from build123d import *

# Parameters (mm, degrees)
F0_W     = 20
F0_H     = 7
F0_H_2   = 62
F0_W_2   = 16
F0_H_3   = 58
F1_DEPTH = 2
F2_DEPTH = 36
F3_W     = 2
F3_H     = 36
F4_DEPTH = 7
F5_W     = 2
F5_H     = 36
F6_DEPTH = 7
F7_W     = 18
F7_H     = 2
F8_DEPTH = 18


with BuildPart() as f1:
    # F0 (on Top) → F1 (new body)
    with BuildSketch(Plane.XY):
        with Locations((8, 63.5)):
            Rectangle(F0_W, F0_H)
        with Locations((8, 29)):
            Rectangle(F0_W, F0_H_2)
        with Locations((8, 29)):
            Rectangle(F0_W_2, F0_H_3, mode=Mode.SUBTRACT)
        with Locations((8, 29)):
            Rectangle(F0_W_2, F0_H_3)
        with Locations((8, -5.5)):
            Rectangle(F0_W, F0_H)
    extrude(amount=-F1_DEPTH)

    # F0 (on Top) → F2 (join)
    with BuildSketch(Plane.XY):
        with Locations((8, 29)):
            Rectangle(F0_W, F0_H_2)
        with Locations((8, 29)):
            Rectangle(F0_W_2, F0_H_3, mode=Mode.SUBTRACT)
    extrude(amount=F2_DEPTH)

    # F3 (on face) → F4 (join)
    with BuildSketch(Plane.XZ.offset(2)):
        with Locations((-1, 18)):
            Rectangle(F3_W, F3_H)
    extrude(amount=F4_DEPTH)

    # F5 (on face) → F6 (join)
    with BuildSketch(Plane(origin=(0, 60, 0), x_dir=(-1, 0, 0), z_dir=(0, 1, 0))):
        with Locations((1, 18)):
            Rectangle(F5_W, F5_H)
    extrude(amount=F6_DEPTH)

    # F7 (on face) → F8 (cut)
    with BuildSketch(Plane.XY.offset(36)):
        with Locations((9, -1)):
            Rectangle(F7_W, F7_H)
    extrude(amount=-F8_DEPTH, mode=Mode.SUBTRACT)


solid = f1.part
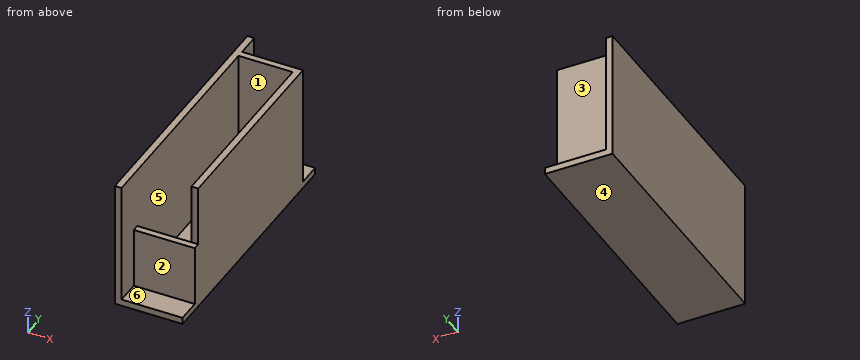
Could you check a few things on this model? Use its own coordinates, in mm. Face numbers are marked on the shaded views. A direction names the side the tool comes from. Round coordinates to 2 decimals unless told otherwise and drop trailing zeros. Write each loop counter-clockwise with the first axis right and the second up, starting at its lowest first coordinate (ties: lowest second). Pieces come first, ordered by that corner, then holes. Notation, with made-up numbers: (3.25, 65.25) - (43.25, 65.25) arc R9 cw to (43.25, 73.25) - close; hole circle Ø3 at (27.25, 68.25). An arc over 180 degrees is marked (long way). Use a Markdown table: item, result.
Q1. Please list where these lines run through material, in increasing order: L1, parallel to X at y = 52, z = 18.5; L2, parallel to Y at x = 7, z = 13; L3, parallel to Y at x = 10.25, z = 19.
Output values:
| item | result |
|---|---|
| L1 | -2 to 0, 16 to 18 |
| L2 | -2 to 0, 58 to 60 |
| L3 | 58 to 60 |
Q2. I want a section at A-A (z = 5.5). List the corners of the cut face in (x, y) for me, plus the area to 3 significant figures.
Output values:
| item | result |
|---|---|
| outline | (-2, -9) - (0, -9) - (0, -2) - (18, -2) - (18, 60) - (0, 60) - (0, 67) - (-2, 67) - close; hole (0, 0) - (16, 0) - (16, 58) - (0, 58) - close |
| area | 340 mm2 |
Q3. Thinking about a two-plate mould opening in Y: for the marked faces 1, 2 and 3, which applies, released by +Y, released by -Y, zero draft, split by the parting line, or undercut?
Output values:
| item | result |
|---|---|
| face 1 | undercut |
| face 2 | released by -Y |
| face 3 | released by +Y |
Q4. I want a section at C-C (x = 7.75). List the corners of the cut face in (y, z) for me, plus the area to 3 significant figures.
Output values:
| item | result |
|---|---|
| outline | (-9, -2) - (67, -2) - (67, 0) - (60, 0) - (60, 36) - (58, 36) - (58, 0) - (0, 0) - (0, 18) - (-2, 18) - (-2, 0) - (-9, 0) - close |
| area | 260 mm2 |
Q5. For the marked faces 4, 5 and 6, which set-ups out of +Z, -Z, +X, -X, +Y, -Y let a thin tool reach every point of the face, with its end or its side?
Output values:
| item | result |
|---|---|
| face 4 | -Z, +X, -X, +Y, -Y |
| face 5 | +Z |
| face 6 | +Z, +X, -Y |
Q6. For pin 1 (5.5 mm diameter, centred on x = 5, y = -5.5, fed in from +Z); pin 2 (5 mm diameter, centred on x = 10, z = 23, fed in from -Y); pin 3 (1.6 mm diameter, centred on x = 17, z = 30, fed in from -Y), each with a flat end and sliding along its axis, tell me the tip position at first contact or that it passes through.
Output values:
| item | result |
|---|---|
| pin 1 | z = 0 |
| pin 2 | y = 58 |
| pin 3 | y = 0 |
Q7. I want a section at B-B (y = 41.5). List the corners of the cut face in (x, z) for me.
Output values:
| item | result |
|---|---|
| outline | (-2, -2) - (18, -2) - (18, 36) - (16, 36) - (16, 0) - (0, 0) - (0, 36) - (-2, 36) - close |
Q8. I want a section at D-D (z = 21). List the corners of the cut face in (x, y) for me, plus the area to 3 significant figures.
Output values:
| item | result |
|---|---|
| outline | (-2, -9) - (0, -9) - (0, 58) - (16, 58) - (16, 0) - (18, 0) - (18, 60) - (0, 60) - (0, 67) - (-2, 67) - close |
| area | 304 mm2 |
